Geometry: final body of the model. Coordinates: model frame, mm. A direction names the side the tool comes from. Round coordinates to 2 decimals unless told otherwise and drop trailing zeros. Write each loop counter-clockwise with the first axis right and the second up, starting at its lowest first coordinate (ties: lowest second). Pieces come first, ordered by that corner, then holes. Notation, with made-up numbers: (4.25, 58) - (33.25, 58) arc R10 ccw to (33.25, 69) - close; hole circle Ø7 at (53, 64). An arc over 180 degrees is marked (long way). Write each question's results on one line, items separated by ' | '.
from build123d import *

# Parameters (mm, degrees)
F0_R     = 1.75
F1_DEPTH = 4


with BuildPart() as f1:
    # F0 (on Top) → F1 (new body)
    with BuildSketch(Plane.XY):
        with BuildLine():
            Line((-15, -8), (-9, -8))
            Line((-9, -8), (-9, -3.5))
            Line((-9, -3.5), (9, -3.5))
            Line((9, -3.5), (9, -8))
            Line((9, -8), (15, -8))
            Line((15, -8), (15, -3.5))
            Line((15, -3.5), (33, -3.5))
            Line((33, -3.5), (33, -8))
            Line((33, -8), (39, -8))
            Line((39, -8), (39, -3.5))
            Line((39, -3.5), (57, -3.5))
            Line((57, -3.5), (57, -8))
            Line((57, -8), (63, -8))
            Line((63, -8), (63, 4))
            Line((63, 4), (-47, 8))
            Line((-47, 8), (-60, 8))
            ThreePointArc((-60, 8), (-62.12132, 7.12132), (-63, 5))
            Line((-63, 5), (-63, -5))
            ThreePointArc((-63, -5), (-62.12132, -7.12132), (-60, -8))
            Line((-60, -8), (-47, -8))
            Line((-47, -8), (-47, -3.5))
            Line((-47, -3.5), (-41, -3.5))
            Line((-41, -3.5), (-41, -8))
            Line((-41, -8), (-33, -8))
            Line((-33, -8), (-33, -3.5))
            Line((-33, -3.5), (-15, -3.5))
            Line((-15, -3.5), (-15, -8))
        make_face()
        with Locations((-55, 0)):
            Circle(F0_R, mode=Mode.SUBTRACT)
    extrude(amount=F1_DEPTH)


solid = f1.part
Q1. Section query A-A, the plane y = 0. Return loops of the section in (x, z), plus the area to 3 significant figures.
Answer block:
outline: (-63, 0) - (-56.75, 0) - (-56.75, 4) - (-63, 4) - close; (-53.25, 0) - (63, 0) - (63, 4) - (-53.25, 4) - close | area: 490 mm2
Q2. Section query B-B, the plane z = 1.2. Return loops of the section in (x, y), plus the area to 3 significant figures.
Answer block:
outline: (-63, -5) arc R3 ccw to (-60, -8) - (-47, -8) - (-47, -3.5) - (-41, -3.5) - (-41, -8) - (-33, -8) - (-33, -3.5) - (-15, -3.5) - (-15, -8) - (-9, -8) - (-9, -3.5) - (9, -3.5) - (9, -8) - (15, -8) - (15, -3.5) - (33, -3.5) - (33, -8) - (39, -8) - (39, -3.5) - (57, -3.5) - (57, -8) - (63, -8) - (63, 4) - (-47, 8) - (-60, 8) arc R3 ccw to (-63, 5) - close; hole circle Ø3.5 at (-55, 0) | area: 1,430 mm2
Q3. Mould query, pull axis X, two halves, no side actions, for faces 3 (the flat face through (-54, -8, 2)), 4 (the flat face through (33, -6, 2)), 5 (the flat face through (-63, 0, 2)). Classes: pulls with the +X half, pulls with the -X half, needs draft (parallel to the pull), parting line crosses it, or undercut.
Answer block:
face 3: needs draft | face 4: undercut | face 5: pulls with the -X half
Q4. Access query for faces 1 (the flat face through (-1, 0, 0)), 2 (the flat face through (24, -3.5, 2)). Directions: +Z, -Z, +X, -X, +Y, -Y. A direction counts if a zero-diameter tool reaches every point of the face in a straight line with its end or side. Return the directions, or none.
Answer block:
face 1: -Z, +X, -X, +Y, -Y | face 2: +Z, -Z, -Y
Q5. Pin query (flat end, axial travel): pin 1 (2 mm diameter, centred on x = 44, z = 2, fed in from -Y); pin 2 (1 mm diameter, centred on x = -19, z = 1.5, fed in from +Y); pin 3 (1.2 mm diameter, centred on y = -7, z = 2.5, fed in from -X). Return the tip coordinate at first contact, or that it passes through.
Answer block:
pin 1: y = -3.5 | pin 2: y = 7 | pin 3: x = -62.65
Q6. Ray query, line 1 along X through (y, z) = (-4.5, 2.4); line 2 along Y through (x, z) = (-55, 3.15); line 3 along Y through (x, z) = (-54, 1.6). Return the intervals inside material, ascending.
Answer block:
line 1: -63 to -47, -41 to -33, -15 to -9, 9 to 15, 33 to 39, 57 to 63 | line 2: -8 to -1.75, 1.75 to 8 | line 3: -8 to -1.44, 1.44 to 8
Q7. Section query D-D, the plane x = -35.5. Return loops of the section in (y, z).
Answer block:
outline: (-8, 0) - (7.58, 0) - (7.58, 4) - (-8, 4) - close
Q8. Section query C-C, the plane x = -55. Return loops of the section in (y, z).
Answer block:
outline: (-8, 0) - (-1.75, 0) - (-1.75, 4) - (-8, 4) - close; (1.75, 0) - (8, 0) - (8, 4) - (1.75, 4) - close
